Geometry check sheet. Reference: the model listing, model coordinates, mm. A direction names the side the tool comes from. Give positions to 0.01 mm unless a question says otherwise; leave off trailing zeros. Loops run counter-clockwise (first coordinate to the right, second up) from the corner with the lowest first, then second, coordinate; pieces in that order, holes last. Notation, with made-up numbers: (86, 55.5) -> (108, 55.5) arc R12 ccw to (108, 75.5) -> close; hole circle Ø1 at (73, -17.75). An arc over 180 degrees is marked (long way). Write item = value, one per line.
```python
from build123d import *

# Parameters (mm, degrees)
BOSS_EXTRUDE1_DEPTH     = 2.54
F_1_4_CLEARANCE_HOLE1_D = 6.7564


with BuildPart() as part:
    # Sketch1 → Boss-Extrude1 (new body)
    with BuildSketch(Plane(origin=(0, 0, 0), x_dir=(0, 0, -1), z_dir=(1, 0, 0))):
        with BuildLine():
            Line((-13.43658162, 13.504102131), (37.36341838, 64.050102131))
            ThreePointArc((37.36341838, 64.050102131), (43.531941304, 68.155026742), (50.8, 69.596))
            Line((50.8, 69.596), (127, 69.596))
            ThreePointArc((127, 69.596), (135.498900621, 67.595081742), (142.212435842, 62.012660183))
            Line((142.212435842, 62.012660183), (180.312435842, 11.466660183))
            ThreePointArc((180.312435842, 11.466660183), (171.145891051, -18.065151574), (146.05, 0))
            ThreePointArc((146.05, 0), (136.82503518, 22.27103518), (114.554, 31.496))
            Line((114.554, 31.496), (50.546, 31.496))
            ThreePointArc((50.546, 31.496), (28.27496482, 22.27103518), (19.05, 0))
            ThreePointArc((19.05, 0), (-7.31216863, -17.590755809), (-13.43658162, 13.504102131))
        make_face()
    extrude(amount=BOSS_EXTRUDE1_DEPTH)

    # 1/4 Clearance Hole1 (through all)
    with Locations(Plane(origin=(2.54, 0, 0), x_dir=(0, 0, -1), z_dir=(1, 0, 0))):
        with Locations((50.8, 50.546), (127, 50.546), (165.1, 0), (0, 0)):
            Hole(F_1_4_CLEARANCE_HOLE1_D / 2)


solid = part.part
```
Item 1: Tool access check on faces 1 (the cylindrical face through (1.252, 22.025, -137.069)), 2 (the cylindrical face through (1.3, 68.1, -43.4)). Record the directions out of +Z, -Z, +X, -X, +Y, -Y that give a thin tool (end or side, any length) a straight path to the whole face; none if there is none.
Answer:
face_1 = +X, -X, -Y
face_2 = +Z, +X, -X, +Y
Item 2: Draft check along Z on faces 3 (the cylindrical face through (1.25, -17.9, -171.62)), 4 (the flat face through (0, 36, -84)), 5 (the flat face through (1.252, 38.423, -11.608)), 6 (the cylindrical face through (1.252, 22.515, -28.521)). Enter one of: +Z half, -Z half, draft (parallel to the pull), parting line (faces both ways), or undercut.
Answer:
face_3 = undercut
face_4 = draft
face_5 = +Z half
face_6 = undercut
Item 3: Thickness scan on L1, parallel to Z at x = 1.45, y = -0.5; L2, parallel to Z at x = 1.35, y = -2; L3, parallel to Y at x = 0.95, z = -63.5. Record the ranges inside material, lowest first. Write a range as [from, to].
Answer:
L1 = [-184.14, -168.44], [-161.76, -146.06], [-19.04, -3.34], [3.34, 19.04]
L2 = [-184.04, -167.82], [-162.38, -146.16], [-18.94, -2.72], [2.72, 18.94]
L3 = [31.5, 69.6]
Item 4: Section check A-A, the plane y = 16. Record the cut outline in (x, z), plus the area to 3 significant figures.
Answer:
outline = (0, -176.9) -> (2.54, -176.9) -> (2.54, -141.68) -> (0, -141.68) -> close; (0, -23.42) -> (2.54, -23.42) -> (2.54, 10.93) -> (0, 10.93) -> close
area = 177 mm^2
Item 5: Gauge pin test, flat ends, axial feed: pin 1 (0.8 mm diameter, centred on x = 2, z = -85.5, fed in from -Y); pin 2 (8 mm diameter, centred on y = 0, z = 0, fed in from +X). Record the tip position at first contact, or that the pin passes through.
Answer:
pin_1 = 31.5
pin_2 = 2.54
Item 6: Section check D-D, the plane z = -151. Record the cut outline in (x, y).
Answer:
outline = (0, -12.81) -> (2.54, -12.81) -> (2.54, 50.35) -> (0, 50.35) -> close
Item 7: Section check C-C, the plane x = 1. Record the cut outline in (y, z).
Answer:
outline = (0, -146.05) arc R19.05 ccw (long way) to (11.47, -180.31) -> (62.01, -142.21) arc R19.05 ccw to (69.6, -127) -> (69.6, -50.8) arc R19.05 ccw to (64.05, -37.36) -> (13.5, 13.44) arc R19.05 ccw (long way) to (0, -19.05) arc R31.5 cw to (31.5, -50.55) -> (31.5, -114.55) arc R31.5 cw to start; hole circle Ø6.76 at (0, -165.1); hole circle Ø6.76 at (0, 0); hole circle Ø6.76 at (50.55, -127); hole circle Ø6.76 at (50.55, -50.8)
Item 8: Section check B-B, the plane z = 1.5. Record the cut outline in (x, y), plus the area to 3 significant figures.
Answer:
outline = (0, -18.99) -> (2.54, -18.99) -> (2.54, -3.03) -> (0, -3.03) -> close; (0, 3.03) -> (2.54, 3.03) -> (2.54, 25.38) -> (0, 25.38) -> close
area = 97.3 mm^2
